Verification items for the finished model (mm, model axes). Round coordinates to 2 decimals unless told otherwise and drop trailing zeros. Write each loop counter-clockwise with the first axis right and the second up, starting at its lowest first coordinate (ties: lowest second). Pieces come first, ordered by that corner, then holes. Notation, with made-up numbers: M 71.25,65 L 105.25,65 A27 ccw 105.25,83 Z; hole C -31,64.5 d2. An arc over 180 degrees is marked long. One line per question, with ' | ' between items.
from build123d import *

# Parameters (mm, degrees)
SKETCH1_W           = 8
SKETCH1_H           = 8
BOSS_EXTRUDE1_DEPTH = 35
SKETCH2_R           = 1.5
CUT_EXTRUDE1_DEPTH  = 37.124783736
SKETCH3_R           = 1.5
CUT_EXTRUDE2_DEPTH  = 37.124783736


with BuildPart() as part:
    # Sketch1 → Boss-Extrude1 (new body)
    with BuildSketch(Plane(origin=(0, 0, 0), x_dir=(1, 0, 0), z_dir=(0, 1, 0))):
        Rectangle(SKETCH1_W, SKETCH1_H)
    extrude(amount=BOSS_EXTRUDE1_DEPTH)

    # Sketch2 → Cut-Extrude1 (cut, through all)
    with BuildSketch(Plane(origin=(0, 0, -4), x_dir=(-1, 0, 0), z_dir=(0, 0, -1))):
        with Locations((0, 31)):
            Circle(SKETCH2_R)
        with Locations((0, 21)):
            Circle(SKETCH2_R)
    extrude(amount=-CUT_EXTRUDE1_DEPTH, mode=Mode.SUBTRACT)

    # Sketch3 → Cut-Extrude2 (cut, through all)
    with BuildSketch(Plane(origin=(4, 0, 0), x_dir=(0, 0, -1), z_dir=(1, 0, 0))):
        with Locations((0, 15)):
            Circle(SKETCH3_R)
        with Locations((0, 5)):
            Circle(SKETCH3_R)
    extrude(amount=-CUT_EXTRUDE2_DEPTH, mode=Mode.SUBTRACT)


solid = part.part
1. Mould release check, pull along Z, two halves, no side actions. Record for faces 1 (the face through (0, 17, -4)), 2 (the face through (-4, 17, 0)), 3 (the face through (0.06, 16.01, 1.11)): pulls with the +Z half, pulls with the -Z half, needs draft (parallel to the pull), parting line crosses it, or undercut.
Results:
face 1: pulls with the -Z half | face 2: needs draft | face 3: undercut
2. Section check B-B, the plane x = 0. Record the cut outline in (y, z), then the cut area to 3 significant figures.
Results:
outline: M 0,-4 L 19.5,-4 L 19.5,4 L 0,4 Z; M 22.5,-4 L 29.5,-4 L 29.5,4 L 22.5,4 Z; M 32.5,-4 L 35,-4 L 35,4 L 32.5,4 Z; hole C 5,0 d3; hole C 15,0 d3 | area: 218 mm2
3. Section check C-C, the plane y = 31. Record the cut outline in (x, z), then the cut area to 3 significant figures.
Results:
outline: M -4,-4 L -1.5,-4 L -1.5,4 L -4,4 Z; M 1.5,-4 L 4,-4 L 4,4 L 1.5,4 Z | area: 40.0 mm2
4. Go/stop test with a flat-tipped pin: P1, Ø3.5, axis at y = 15, z = 0, coming from the -X side. Record where the tip stops, or that it passes through.
Results:
P1: stops at x = -4
5. Thickness scan on line 1 (Y direction, x = -2, z = 0); line 2 (Y direction, x = 0, z = 2); line 3 (Y direction, x = 0, z = -0.5). Record the ranges inside material, lowest first.
Results:
line 1: y = 0 to 3.5, 6.5 to 13.5, 16.5 to 35 | line 2: y = 0 to 19.5, 22.5 to 29.5, 32.5 to 35 | line 3: y = 0 to 3.59, 6.41 to 13.59, 16.41 to 19.5, 22.5 to 29.5, 32.5 to 35
6. Section check A-A, the plane z = 0. Record the cut outline in (x, y), then the cut area to 3 significant figures.
Results:
outline: M -4,0 L 4,0 L 4,3.5 L -4,3.5 Z; M -4,6.5 L 4,6.5 L 4,13.5 L -4,13.5 Z; M -4,16.5 L 4,16.5 L 4,35 L -4,35 Z; hole C 0,21 d3; hole C 0,31 d3 | area: 218 mm2
7. Section check D-D, the plane z = 2.25. Record the cut outline in (x, y).
Results:
outline: M -4,0 L 4,0 L 4,35 L -4,35 Z; hole C 0,21 d3; hole C 0,31 d3
